Source: CAD feature listing. Evaluate the final solid. Frame: model axes, mm. Face numbers are marked on the shaded views. Round coordinates to 2 decimals unless told otherwise and drop trailing zeros. Loops run counter-clockwise (first coordinate to the right, second up) from the corner with the lowest first, then second, coordinate; pieces in that order, holes last. Notation, with made-up numbers: M 82,84.25 L 99,84.25 A30 ccw 99,121.25 Z; hole C -22,79.5 d3. An arc over 180 degrees is marked long. One line per item, written item: value.
from build123d import *

# Parameters (mm, degrees)
EXTRUDE_THIN1_DEPTH = 219.218052
CUT_EXTRUDE1_DEPTH  = 223.141563699


with BuildPart() as part:
    # Sketch1 → Extrude-Thin1 (new body)
    with BuildSketch(Plane.XY):
        with BuildLine():
            Line((-12.7, 22.86), (-12.7, -22.86))
            ThreePointArc((-12.7, -22.86), (-11.956051224, -24.656051224), (-10.16, -25.4))
            Line((-10.16, -25.4), (10.16, -25.4))
            ThreePointArc((10.16, -25.4), (11.956051224, -24.656051224), (12.7, -22.86))
            Line((12.7, -22.86), (12.7, 22.86))
            ThreePointArc((12.7, 22.86), (11.956051224, 24.656051224), (10.16, 25.4))
            Line((10.16, 25.4), (-10.16, 25.4))
            ThreePointArc((-10.16, 25.4), (-11.956051224, 24.656051224), (-12.7, 22.86))
        make_face()
        with BuildLine():
            Line((-11.1125, 22.86), (-11.1125, -22.86))
            ThreePointArc((-11.1125, -22.86), (-10.833519209, -23.533519209), (-10.16, -23.8125))
            Line((-10.16, -23.8125), (10.16, -23.8125))
            ThreePointArc((10.16, -23.8125), (10.833519209, -23.533519209), (11.1125, -22.86))
            Line((11.1125, -22.86), (11.1125, 22.86))
            ThreePointArc((11.1125, 22.86), (10.833519209, 23.533519209), (10.16, 23.8125))
            Line((10.16, 23.8125), (-10.16, 23.8125))
            ThreePointArc((-10.16, 23.8125), (-10.833519209, 23.533519209), (-11.1125, 22.86))
        make_face(mode=Mode.SUBTRACT)
    extrude(amount=EXTRUDE_THIN1_DEPTH)

    # Sketch2 → Cut-Extrude1 (cut, through all)
    with BuildSketch(Plane(origin=(12.7, 0, 0), x_dir=(0, 0, -1), z_dir=(1, 0, 0))):
        Polygon((-219.218051789, 25.4), (-176.591790525, -25.4), (-219.218051789, -25.4), align=None)
        Polygon((0, 25.4), (-60.541082504, -25.4), (0, -25.4), align=None)
    extrude(amount=-CUT_EXTRUDE1_DEPTH, mode=Mode.SUBTRACT)


solid = part.part
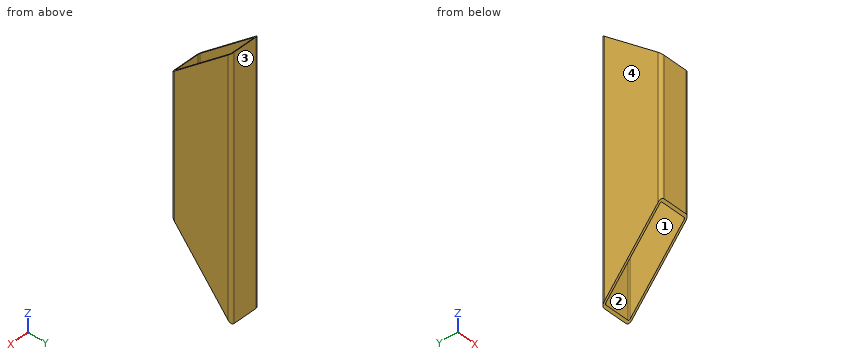
1. Pull-direction query (Y, two-part tool) for the marked faces 1, 2, 3 and 4; classes: released by +Y, released by -Y, zero draft, split by the parting line, or undercut.
Report:
face 1: undercut
face 2: undercut
face 3: released by +Y
face 4: zero draft
2. Section query B-B (y = 11). Return the cut outline in (x, z).
Report:
outline: M -12.7,17.16 L -11.11,17.16 L -11.11,207.14 L -12.7,207.14 Z; M 11.11,17.16 L 12.7,17.16 L 12.7,207.14 L 11.11,207.14 Z
3. Ray query, line 1 (X direction, y = 13, z = 87); line 2 (Y direction, x = -9, z = 107); line 3 (Y direction, x = -9, z = 199). Return the intervals inside material, ascending. Write a range as [from, to].
Report:
line 1: x = [-12.7, -11.11], [11.11, 12.7]
line 2: y = [-25.4, -23.81], [23.81, 25.4]
line 3: y = [23.81, 25.4]
4. Section query D-D (z = 191.5). Return the cut outline in (x, y) (1 decimal), and give its area (3 significant figures).
Report:
outline: M -12.7,-7.6 L -11.1,-7.6 L -11.1,22.9 A1 cw -10.2,23.8 L 10.2,23.8 A1 cw 11.1,22.9 L 11.1,-7.6 L 12.7,-7.6 L 12.7,22.9 A2.5 ccw 10.2,25.4 L -10.2,25.4 A2.5 ccw -12.7,22.9 Z
area: 138 mm2
5. Section query A-A (x = -8). Return the cut outline in (y, z), and give its area (3 significant figures).
Report:
outline: M -25.4,60.54 L -23.81,58.65 L -23.81,177.92 L -25.4,176.59 Z; M 23.81,1.89 L 25.4,0 L 25.4,219.22 L 23.81,217.89 Z
area: 532 mm2
6. Section query C-C (z = 160). Return the cut outline in (x, y) (1 decimal), and give its area (3 significant figures).
Report:
outline: M -12.7,-22.9 A2.5 ccw -10.2,-25.4 L 10.2,-25.4 A2.5 ccw 12.7,-22.9 L 12.7,22.9 A2.5 ccw 10.2,25.4 L -10.2,25.4 A2.5 ccw -12.7,22.9 Z; hole M -11.1,-22.9 A1 ccw -10.2,-23.8 L 10.2,-23.8 A1 ccw 11.1,-22.9 L 11.1,22.9 A1 ccw 10.2,23.8 L -10.2,23.8 A1 ccw -11.1,22.9 Z
area: 227 mm2
7. Pin query (flat end, axial travel): pin 1 (10 mm diameter, centred on x = 3.5, y = 0, fed in from +Z). Return the tip coordinate at first contact, or that it passes through.
Report:
pin 1: passes through
